For this review, take the finished solid that the model builds, in its own axes (mm). A direction names the side the tool comes from. Coordinates: 2 decimals unless noted, no trailing zeros. Loops run counter-clockwise (first coordinate to the right, second up) from the corner with the lowest first, then second, coordinate; pieces in that order, holes last. Notation, with made-up numbers: (74.5, 29.25) -> (116.5, 29.25) arc R25 cw to (116.5, 57.25) -> close; hole circle Ø2 at (78.25, -1.75). An arc over 180 degrees is marked (long way). Answer in a Markdown table with one row per item.
from build123d import *

# Parameters (mm, degrees)
SKETCH1_W           = 10
SKETCH1_H           = 10
SKETCH1_R           = 2.05
BOSS_EXTRUDE1_DEPTH = 6
CUT_EXTRUDE1_DEPTH  = 3.2
SKETCH3_W           = 10
SKETCH3_H           = 6
BOSS_EXTRUDE2_DEPTH = 20
SKETCH4_R           = 2.05
CUT_EXTRUDE2_DEPTH  = 27.191601707
CUT_EXTRUDE3_DEPTH  = 3.2
SKETCH6_R           = 2.2
BOSS_EXTRUDE3_DEPTH = 4.5
SKETCH7_W           = 10
SKETCH7_H           = 10.114722763
CUT_EXTRUDE4_DEPTH  = 1.6


with BuildPart() as part:
    # Sketch1 → Boss-Extrude1 (new body)
    with BuildSketch(Plane(origin=(0, 0, 0), x_dir=(1, 0, 0), z_dir=(0, 1, 0))):
        Rectangle(SKETCH1_W, SKETCH1_H)
        with Locations(Location((0, 0, 0), (0, 0, 270))):
            Circle(SKETCH1_R, mode=Mode.SUBTRACT)
    extrude(amount=BOSS_EXTRUDE1_DEPTH)

    # Sketch2 → Cut-Extrude1 (cut)
    with BuildSketch(Plane(origin=(0, 6, 0), x_dir=(1, 0, 0), z_dir=(0, 1, 0))):
        Polygon((4.041451884, 0), (2.020725942, 3.5), (-2.020725942, 3.5), (-4.041451884, 0), (-2.020725942, -3.5), (2.020725942, -3.5), align=None)
    extrude(amount=-CUT_EXTRUDE1_DEPTH, mode=Mode.SUBTRACT)

    # Sketch3 → Boss-Extrude2 (add)
    with BuildSketch(Plane(origin=(5, 0, 0), x_dir=(0, 0, -1), z_dir=(1, 0, 0))):
        with Locations((0, 3)):
            Rectangle(SKETCH3_W, SKETCH3_H)
    extrude(amount=BOSS_EXTRUDE2_DEPTH)

    # Sketch4 → Cut-Extrude2 (cut, through all)
    with BuildSketch(Plane(origin=(0, 6, 0), x_dir=(1, 0, 0), z_dir=(0, 1, 0))):
        with Locations(Location((20, 0, 0), (0, 0, 270))):
            Circle(SKETCH4_R)
    extrude(amount=-CUT_EXTRUDE2_DEPTH, mode=Mode.SUBTRACT)

    # Sketch5 → Cut-Extrude3 (cut)
    with BuildSketch(Plane(origin=(0, 6, 0), x_dir=(1, 0, 0), z_dir=(0, 1, 0))):
        Polygon((24.041451884, 0), (22.020725942, 3.5), (17.979274058, 3.5), (15.958548116, 0), (17.979274058, -3.5), (22.020725942, -3.5), align=None)
    extrude(amount=-CUT_EXTRUDE3_DEPTH, mode=Mode.SUBTRACT)

    # Sketch6 → Boss-Extrude3 (add, symmetric)
    with BuildSketch(Plane.ZY.offset(-10)):
        with BuildLine():
            Line((5, 6), (5, 11))
            ThreePointArc((5, 11), (0, 16), (-5, 11))
            Line((-5, 11), (-5, 6))
            Line((-5, 6), (5, 6))
        make_face()
        with Locations((0, 11)):
            Circle(SKETCH6_R, mode=Mode.SUBTRACT)
    extrude(amount=BOSS_EXTRUDE3_DEPTH, both=True)

    # Sketch7 → Cut-Extrude4 (cut, symmetric)
    with BuildSketch(Plane.ZY.offset(-10)):
        with Locations((0, 11.057361381)):
            Rectangle(SKETCH7_W, SKETCH7_H)
    extrude(amount=CUT_EXTRUDE4_DEPTH, both=True, mode=Mode.SUBTRACT)


solid = part.part
Item 1: For L1, parallel to X at y = 2.1, z = 0; L2, parallel to X at y = 9.75, z = -2.5; L3, parallel to Z at x = 13.1, y = 11, list the stretches that pass through material, from the lowest coordinate up.
Worked answers:
| item | result |
|---|---|
| L1 | -5 to -2.05, 2.05 to 17.95, 22.05 to 25 |
| L2 | 5.5 to 8.4, 11.6 to 14.5 |
| L3 | -5 to -2.2, 2.2 to 5 |
Item 2: Take a section at D-D, the plane z = -1. Count the separate pieces of the cut face and the enclosed holes in it, and give its area (3 significant figures).
Worked answers:
| item | result |
|---|---|
| separate pieces | 5 |
| enclosed holes | 0 |
| area | 150 mm² |
Item 3: Insertion check: pin 1 (6 mm diameter, centred on y = 11, z = 2.5, fed in from -X); pin 2 (2 mm diameter, centred on y = 14.5, z = 2, fed in from +X). Each pin has a flat end and moves straight along its axis. Give the tip position at first contact, or say it passes through.
Worked answers:
| item | result |
|---|---|
| pin 1 | x = 5.5 |
| pin 2 | x = 14.5 |
Item 4: Take a section at C-C, the plane y = 3.25. State the section outline as (x, z) points.
Worked answers:
| item | result |
|---|---|
| outline | (-5, -5) -> (25, -5) -> (25, 5) -> (-5, 5) -> close; hole (-4.04, 0) -> (-2.02, -3.5) -> (2.02, -3.5) -> (4.04, 0) -> (2.02, 3.5) -> (-2.02, 3.5) -> close; hole (15.96, 0) -> (17.98, -3.5) -> (22.02, -3.5) -> (24.04, 0) -> (22.02, 3.5) -> (17.98, 3.5) -> close |
Item 5: Take a section at B-B, the plane y = 8. State the section outline as (x, z) points.
Worked answers:
| item | result |
|---|---|
| outline | (5.5, -5) -> (8.4, -5) -> (8.4, 5) -> (5.5, 5) -> close; (11.6, -5) -> (14.5, -5) -> (14.5, 5) -> (11.6, 5) -> close |
Item 6: For faces 1 (the flat face through (20, 4, -3.5)), 2 (the flat face through (11.6, 8.8, 1)), 3 (the flat face through (14.5, 8.8, 1)), list the 3-axis set-ups (+Z, -Z, +X, -X, +Y, -Y) from which the entire face can be reached by the end or side of a thin tool; tool diameter is ignored.
Worked answers:
| item | result |
|---|---|
| face 1 | +Y |
| face 2 | +Z, -Z, +Y |
| face 3 | +Z, -Z, +X, +Y |
Item 7: The part is to be moulded in two halves that separate along X. For faces 4 (the flat face through (10, 4, -5)), 5 (the flat face through (5.5, 8.8, 1)), 6 (the cylindrical face through (2.033, 1.38, -0.267)), say which applies: +X half, -X half, draft (parallel to the pull), parting line (faces both ways), or undercut.
Worked answers:
| item | result |
|---|---|
| face 4 | draft |
| face 5 | -X half |
| face 6 | undercut |
Item 8: Take a section at A-A, the plane x = 0. State the section outline as (y, z) points.
Worked answers:
| item | result |
|---|---|
| outline | (0, -5) -> (6, -5) -> (6, -3.5) -> (2.8, -3.5) -> (2.8, -2.05) -> (0, -2.05) -> close; (0, 2.05) -> (2.8, 2.05) -> (2.8, 3.5) -> (6, 3.5) -> (6, 5) -> (0, 5) -> close |
